Build history of the part. All positions in model axes, mm. Face numbers are marked on the shaded views. A direction names the side the tool comes from. Round coordinates to 2 decimals unless told otherwise and drop trailing zeros. Write each loop counter-clockwise with the first axis right and the second up, starting at its lowest first coordinate (ties: lowest second). Pieces come first, ordered by that corner, then holes.
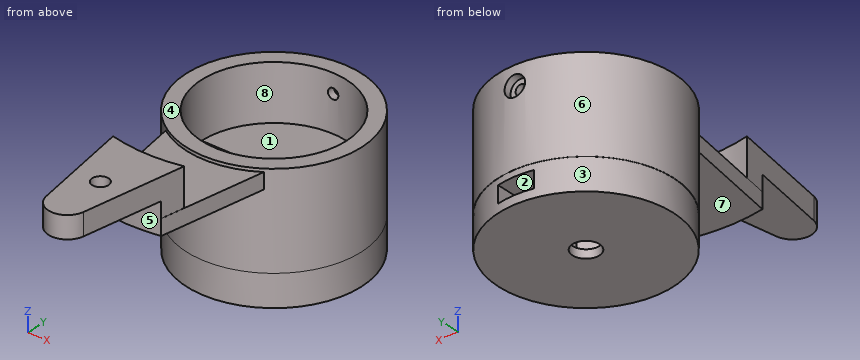
from build123d import *

# Parameters (mm, degrees)
CYLINDER016_R     = 1.65
CYLINDER016_DEPTH = 50
CYLINDER017_R     = 3.25
CYLINDER017_DEPTH = 2.5
BOX005_W          = 80
BOX005_H          = 100
BOX005_DEPTH      = 9.5
CYLINDER014_R     = 22.95
CYLINDER014_DEPTH = 27
CYLINDER015_R     = 27.75
CYLINDER015_DEPTH = 40
SKETCH013_R       = 27.75
PAD001_DEPTH      = 10
SKETCH014_W       = 24
SKETCH014_H       = 14.2
POCKET013_DEPTH   = 28
SKETCH015_R       = 8.1
POCKET014_DEPTH   = 15
POCKET015_DEPTH   = 14.4
PAD003_DEPTH      = 5
PAD004_DEPTH      = 12
POCKET017_DEPTH   = 10
SKETCH033_R       = 2.6
POCKET029_DEPTH   = 4.2
SKETCH034_W       = 108.293205
SKETCH034_H       = 87.132465
POCKET030_DEPTH   = 20
SKETCH035_R       = 27.699707
PAD005_DEPTH      = 10
SKETCH036_W       = 11.3
SKETCH036_H       = 5.3
POCKET031_DEPTH   = 33
POCKET032_DEPTH   = 5.3
SKETCH038_R       = 4.253317
POCKET033_DEPTH   = 8


with BuildPart() as cylinder016:
    # Cylinder016 → Cylinder016 (new body)
    with BuildSketch(Plane(origin=(0, 50, 20), x_dir=(1, 0, 0), z_dir=(0, -1, 0))):
        Circle(CYLINDER016_R)
    extrude(amount=CYLINDER016_DEPTH)


with BuildPart() as cylinder017:
    # Cylinder017 → Cylinder017 (new body)
    with BuildSketch(Plane(origin=(0, 27.75, 20), x_dir=(1, 0, 0), z_dir=(0, -1, 0))):
        Circle(CYLINDER017_R)
    extrude(amount=CYLINDER017_DEPTH)


with BuildPart() as obj1:
    # Box005 → Box005 (new body)
    with BuildSketch(Plane(origin=(-40, 0, -1), x_dir=(1, 0, 0), z_dir=(0, 0, 1))):
        with Locations((40, 50)):
            Rectangle(BOX005_W, BOX005_H)
    extrude(amount=BOX005_DEPTH)


with BuildPart() as fusion007:
    # Cylinder014 → Cylinder014 (new body)
    with BuildSketch(Plane.XY.offset(-1)):
        Circle(CYLINDER014_R)
    extrude(amount=CYLINDER014_DEPTH)

    # Cut011: cut obj1
    add(obj1.part, mode=Mode.SUBTRACT)

    # Fusion007: union Cylinder016, Cylinder017
    add(cylinder016.part)
    add(cylinder017.part)


with BuildPart() as obj2:
    # Cylinder015 → Cylinder015 (new body)
    with BuildSketch(Plane.XY.offset(-14)):
        Circle(CYLINDER015_R)
    extrude(amount=CYLINDER015_DEPTH)

    # Cut010: cut Fusion007
    add(fusion007.part, mode=Mode.SUBTRACT)

    # Sketch013 (on Face2 of BaseFeature003) → Pad001 (new body)
    with BuildSketch(Plane(origin=(0, 0, -14), x_dir=(1, 0, 0), z_dir=(0, 0, -1))):
        Circle(SKETCH013_R)
    extrude(amount=PAD001_DEPTH)

    # Sketch014 → Pocket013 (cut)
    with BuildSketch(Plane(origin=(0, 28, 0), x_dir=(-1, 0, 0), z_dir=(0, 1, 0))):
        with Locations((0, -12.1)):
            Rectangle(SKETCH014_W, SKETCH014_H)
    extrude(amount=-POCKET013_DEPTH, mode=Mode.SUBTRACT)

    # Sketch015 (on Face6 of Pocket013) → Pocket014 (cut)
    with BuildSketch(Plane(origin=(0, 0, -24), x_dir=(1, 0, 0), z_dir=(0, 0, -1))):
        Circle(SKETCH015_R)
    extrude(amount=-POCKET014_DEPTH, mode=Mode.SUBTRACT)

    # Sketch016 (on Face6 of Pocket014) → Pocket015 (cut)
    with BuildSketch(Plane(origin=(0, 0, -19.3), x_dir=(1, 0, 0), z_dir=(0, 0, -1))):
        Polygon((0, -14.036056), (12.155581, -7.018028), (12.155581, 7.018028), (0, 14.036056), (-12.155581, 7.018028), (-12.155581, -7.018028), align=None)
    extrude(amount=-POCKET015_DEPTH, mode=Mode.SUBTRACT)

    # Sketch019 (on Face8 of Pocket015) → Pad003 (join)
    with BuildSketch(Plane.XY.offset(25)):
        with BuildLine():
            ThreePointArc((-15.553331, -22.846971), (0.028426, -27.638548), (15.600294, -22.814929))
            Line((15.600294, -22.814929), (5.918583, -80.985076))
            ThreePointArc((-5.919268, -80.980951), (-0.002091, -86), (5.918583, -80.985076))
            Line((-15.553331, -22.846971), (-5.919268, -80.980951))
        make_face()
    extrude(amount=-PAD003_DEPTH)

    # Sketch031 (on Face12 of Pad003) → Pad004 (join)
    with BuildSketch(Plane.XY.offset(25)):
        with BuildLine():
            ThreePointArc((-5.898869, -81.096969), (0.071542, -85.999573), (5.92335, -80.955994))
            Line((11.272496, -48.593121), (5.92335, -80.955994))
            ThreePointArc((-11.235042, -48.601794), (0.019223, -49.883466), (11.272496, -48.593121))
            Line((-11.235042, -48.601794), (-5.898869, -81.096969))
        make_face()
    extrude(amount=PAD004_DEPTH)

    # Sketch032 (on Face10 of Pad004) → Pocket017 (cut)
    with BuildSketch(Plane(origin=(0, 0, 20), x_dir=(1, 0, 0), z_dir=(0, 0, -1))):
        with BuildLine():
            ThreePointArc((17.426701, 54.194258), (-0.181494, 56.926923), (-17.771906, 54.082038))
            Line((-17.771906, 54.082038), (-17.771906, 91.276634))
            Line((17.426701, 91.276634), (-17.771906, 91.276634))
            Line((17.426701, 54.194258), (17.426701, 91.276634))
        make_face()
    extrude(amount=-POCKET017_DEPTH, mode=Mode.SUBTRACT)

    # Sketch033 (on Face33 of Pocket017) → Pocket029 (cut)
    with BuildSketch(Plane.XY.offset(37)):
        with Locations((0, -67.25)):
            Circle(SKETCH033_R)
    extrude(amount=-POCKET029_DEPTH, mode=Mode.SUBTRACT)

    # Sketch034 (on Face6 of Pocket029) → Pocket030 (cut)
    with BuildSketch(Plane(origin=(0, 0, -24), x_dir=(1, 0, 0), z_dir=(0, 0, -1))):
        with Locations((-3.019794, 5.274049)):
            Rectangle(SKETCH034_W, SKETCH034_H)
    extrude(amount=-POCKET030_DEPTH, mode=Mode.SUBTRACT)

    # Sketch035 (on Face2 of Pocket030) → Pad005 (join)
    with BuildSketch(Plane(origin=(0, 0, -4), x_dir=(1, 0, 0), z_dir=(0, 0, -1))):
        Circle(SKETCH035_R)
    extrude(amount=PAD005_DEPTH)

    # Sketch036 → Pocket031 (cut)
    with BuildSketch(Plane.XZ.offset(-33)):
        with Locations((0, -8.627069)):
            Rectangle(SKETCH036_W, SKETCH036_H)
    extrude(amount=POCKET031_DEPTH, mode=Mode.SUBTRACT)

    # Sketch037 → Pocket032 (cut)
    with BuildSketch(Plane.XY.offset(-6)):
        Polygon((5.65, -3.262029), (5.65, 3.262029), (0, 6.524058), (-5.65, 3.262029), (-5.65, -3.262029), (0, -6.524058), align=None)
    extrude(amount=-POCKET032_DEPTH, mode=Mode.SUBTRACT)

    # Sketch038 (on Face16 of Pocket032) → Pocket033 (cut)
    with BuildSketch(Plane(origin=(0, 0, -14), x_dir=(1, 0, 0), z_dir=(0, 0, -1))):
        Circle(SKETCH038_R)
    extrude(amount=-POCKET033_DEPTH, mode=Mode.SUBTRACT)


with BuildPart() as obj2_1:
    # Body003 placement: moved
    add(obj2.part.moved(Location((0, 0, -67.7))))


solid = obj2_1.part
1) Pin check, flat tips, straight feed: pin 1 Ø2 at (x, z) = (0, -47.7) entering from +Y; pin 2 Ø12.5 at (x, y) = (2, 15.5) entering from +Z; pin 3 Ø6 at (x, z) = (0, -47.7) entering from +Y; pin 4 Ø8 at (x, y) = (-14, -53.5) entering from +Z. Stop position of each tip, or through.
Results:
pin 1: stops at y = -22.93
pin 2: stops at z = -59.2
pin 3: stops at y = 25.25
pin 4: stops at z = -30.7
2) Wall check: L1, parallel to Z at x = 0, y = 24; L2, parallel to Y at x = 0, z = -32.3; L3, parallel to Y at x = 0, z = -61. Give the ranges that are in metal, low to high.
Results:
L1: z = -81.7 to -78.98, -73.68 to -49.35, -46.05 to -41.7
L2: y = -86 to -69.85, -64.65 to -49.88
L3: y = -27.75 to -22.95, 0 to 27.75
3) Slice it at D-D (z = -77.5). Write the cut outline in (x, y).
Results:
outline: (-5.65, -3.26) - (-5.65, 27.12) arc R27.7 ccw (long way) to (5.65, 27.12) - (5.65, -3.26) - (0, -6.52) - close
4) Slice it at C-C (z = -63). Write the cut outline in (x, y), plus the area to 3 significant figures.
Results:
outline: circle Ø55.5 at (0, 0); hole (-22.95, 0) arc R22.95 ccw to (22.95, 0) - close
area: 1,590 mm2
5) Slice it at A-A (x = -21). Write the cut outline in (y, z).
Results:
outline: (-18.14, -71.7) - (-18.06, -71.7) - (-18.06, -81.7) - (18.06, -81.7) - (18.06, -71.7) - (18.14, -71.7) - (18.14, -41.7) - (9.26, -41.7) - (9.26, -59.2) - (0, -59.2) - (0, -68.7) - (-9.26, -68.7) - (-9.26, -41.7) - (-18.14, -41.7) - close
6) Which spindle directions (+Z, -Z, +X, -X, +Y, -Y) get a long thin tool onto all of the face, cutting with end or side? Do the marked faces 1, 2, 3, 4 and 5. Say none if no direction does.
Results:
face 1: +Z
face 2: +Y
face 3: -Z
face 4: +Z, +X, -X, +Y
face 5: -Z, -Y
7) Mould opens along X. For the marked faces 6, 7 and 8 say: released by +X, released by -X, zero draft, split by the parting line, or undercut.
Results:
face 6: split by the parting line
face 7: zero draft
face 8: undercut
